Could you check a few things on this drawing? It's one solid part, dimensions in mm from its lowest x, y, z. A direction names the side the tool comes from. Round coordinates to 2 decimals unless told otherwise and drop trailing zeros. Loops run counter-clockwise (first coordinate to the right, second up) from the corner with the lowest first, then second, coordinate; pieces in that order, holes last. Notation, with made-up numbers: M 51,47 L 62,47 A8 ccw 62,53 Z; hole C 50,80 d9. An arc over 180 degrees is marked long. Return JSON: item names as keys, results as strings.
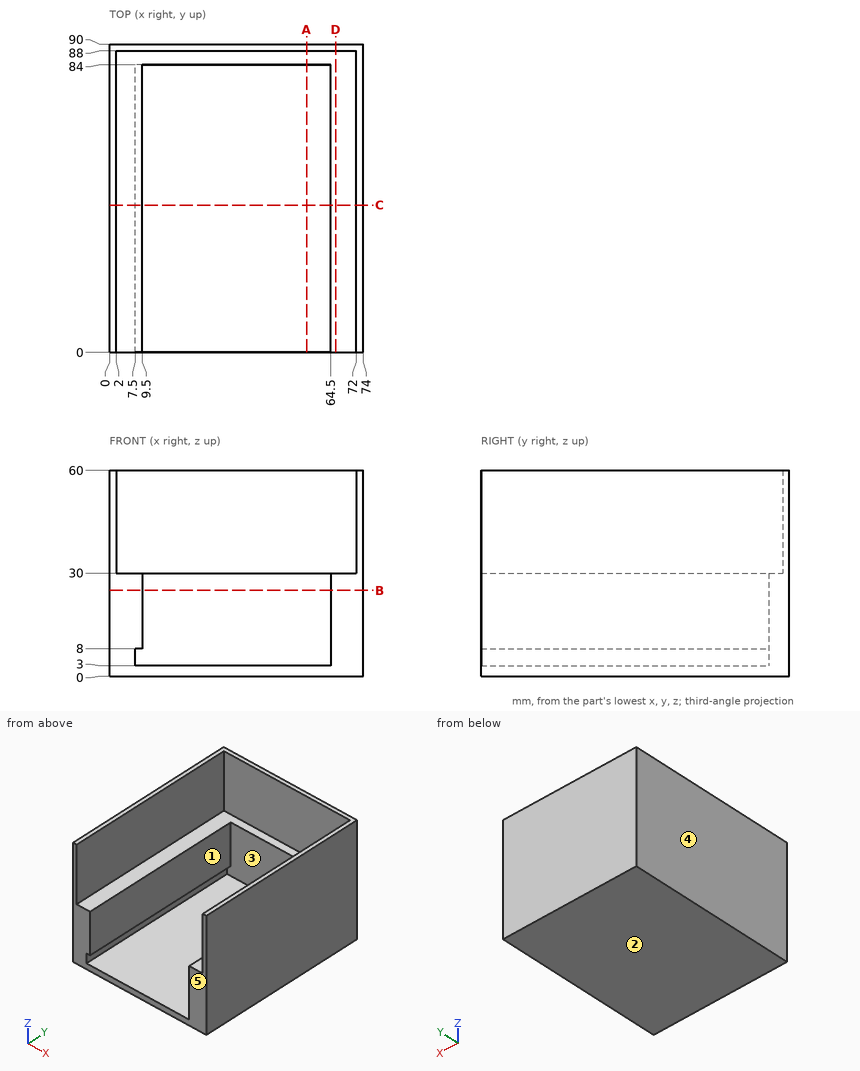
Q1. I'm going to push flat-ended pins straight in: pin 1 Ø6 at (x, y) = (17.5, 49) entering from +Z; pin 2 Ø13.5 at (x, z) = (28, 22.5) entering from -Y; pin 3 Ø9 at (x, z) = (50, 51) entering from -Y. Where does each tip first touch, or does it pass through?
Results:
{"pin 1": "stops at z = 3", "pin 2": "stops at y = 84", "pin 3": "stops at y = 88"}
Q2. Thinking about a two-plate mould opening in X: for the marked faces 3, 4 and 5, which applies, pulls with the +X half, pulls with the -X half, needs draft (parallel to the pull), parting line crosses it, or undercut?
Results:
{"face 3": "undercut", "face 4": "pulls with the -X half", "face 5": "needs draft"}
Q3. Suppose I cut it at C-C, the plane y = 43. Please give me the cut outline in (x, z).
Results:
{"outline": "M 0,0 L 74,0 L 74,60 L 72,60 L 72,30 L 64.5,30 L 64.5,3 L 7.5,3 L 7.5,8 L 9.5,8 L 9.5,30 L 2,30 L 2,60 L 0,60 Z"}
Q4. Suppose I cut it at B-B, the plane z = 25. Please give me the cut outline in (x, y).
Results:
{"outline": "M 0,0 L 9.5,0 L 9.5,84 L 64.5,84 L 64.5,0 L 74,0 L 74,90 L 0,90 Z"}
Q5. Suppose I cut it at D-D, the plane x = 66. Please give me the cut outline in (y, z), plus the area to 3 significant figures.
Results:
{"outline": "M 0,0 L 90,0 L 90,60 L 88,60 L 88,30 L 0,30 Z", "area": "2,760 mm2"}
Q6. If I drill on line 1 along X through (y, z) = (66.5, 25.5); line 2 along X through (y, z) = (85.5, 42); line 3 along Z through (x, y) = (22.5, 85), over which ranges is the centre line in solid material (lowest first)?
Results:
{"line 1": "x = 0 to 9.5, 64.5 to 74", "line 2": "x = 0 to 2, 72 to 74", "line 3": "z = 0 to 30"}
Q7. On a 3-axis mill with a long thin cutter (end or side, diameter ignored), from which of +Z, -Z, +X, -X, +Y, -Y can I reach the whole of each face in a straight line? I mean the marked faces 1 and 2. Say none if no direction works.
Results:
{"face 1": "+Z, -Y", "face 2": "-Z, +X, -X, +Y, -Y"}
Q8. Suppose I cut it at A-A, the plane x = 57.5. Please give me the cut outline in (y, z).
Results:
{"outline": "M 0,0 L 90,0 L 90,60 L 88,60 L 88,30 L 84,30 L 84,3 L 0,3 Z"}
